Here's how the part is built. I have some questions about the finished solid (model axes, mm). Face numbers are marked on the shaded views. A direction names the side the tool comes from. Give positions to 0.01 mm unless a question says otherwise; leave off trailing zeros. Write each loop counter-clockwise with the first axis right and the second up, starting at its lowest first coordinate (ties: lowest second). Pieces come first, ordered by that corner, then holes. Notation, with made-up numbers: (42.5, 6.25) - (77.5, 6.25) arc R30 ccw to (77.5, 45.25) - close; hole circle Ø10 at (-17.75, 35.25). An arc over 180 degrees is marked (long way). Use a Markdown table: item, result.
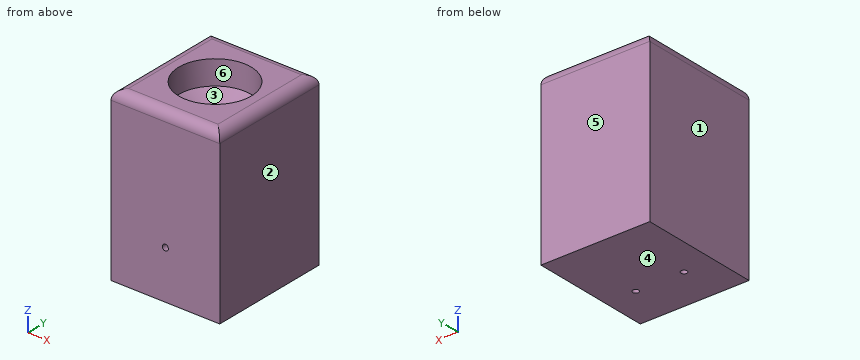
```python
from build123d import *

# Parameters (mm, degrees)
F0_W     = 57.15
F0_H     = 63.5
F1_DEPTH = 88.9
F3_D     = 38.1
F3_DEPTH = 12.7
F3_TIP   = 11.4463947925
F4_R     = 5.08
F6_D     = 3.175
F6_DEPTH = 12.7
F6_TIP   = 0.9538662327
F8_D     = 3.175


with BuildPart() as f1:
    # F0 (on Top) → F1 (new body)
    with BuildSketch(Plane.XY):
        with Locations((28.575, -31.75)):
            Rectangle(F0_W, F0_H)
    extrude(amount=F1_DEPTH)

    # F3
    with Locations(Plane.XY.offset(88.9)):
        with Locations((28.575, -31.75)):
            Hole(F3_D / 2, depth=F3_DEPTH)
            with Locations((0, 0, -(F3_DEPTH + F3_TIP / 2))):  # 118° drill point
                Cone(0, F3_D / 2, F3_TIP, mode=Mode.SUBTRACT)

    # F4
    f4_edges = [f1.edges().sort_by_distance(p)[0] for p in [
        (57.15, -31.75, 88.9),
        (28.575, 0, 88.9),
        (0, -31.75, 88.9),
        (28.575, -63.5, 88.9),
    ]]
    fillet(f4_edges, radius=F4_R)

    # F6
    with Locations(Plane.XZ.offset(63.5)):
        with Locations((28.575, 25.4)):
            Hole(F6_D / 2, depth=F6_DEPTH)
            with Locations((0, 0, -(F6_DEPTH + F6_TIP / 2))):  # 118° drill point
                Cone(0, F6_D / 2, F6_TIP, mode=Mode.SUBTRACT)

    # F8 (through all)
    with Locations(Plane(origin=(0, 0, 0), x_dir=(1, 0, 0), z_dir=(0, 0, -1))):
        with Locations((41.275, 41.275), (15.875, 41.275)):
            Hole(F8_D / 2)


solid = f1.part
```
Item 1: I need wall thicknesses on line 1 along X through (y, z) = (-57.5, 25.4); line 2 along X through (y, z) = (-31, 79); line 3 along X through (y, z) = (-40.5, 6). Which ranges of each line are inside material? Lowest first, please. Write a range as [from, to].
Values:
| item | result |
|---|---|
| line 1 | x = [0, 26.99], [30.16, 57.15] |
| line 2 | x = [0, 9.54], [47.61, 57.15] |
| line 3 | x = [0, 14.49], [17.26, 39.89], [42.66, 57.15] |
Item 2: If we section it at A-A, the plane z = 77.5: Write out the boundary of the cut face in (x, y) (3 decimals).
Values:
| item | result |
|---|---|
| outline | (0, -63.5) - (57.15, -63.5) - (57.15, 0) - (0, 0) - close; hole circle Ø38.1 at (28.575, -31.75) |
Item 3: For the marked faces 5 and 6, which set-ups out of +Z, -Z, +X, -X, +Y, -Y let a thin tool reach every point of the face, with its end or its side?
Values:
| item | result |
|---|---|
| face 5 | +Z, -Z, +X, -X, +Y |
| face 6 | +Z |
Item 4: Thinking about a two-plate mould opening in X: for the marked faces 1, 2, 3 and 4, which applies, +X half, -X half, draft (parallel to the pull), parting line (faces both ways), or undercut?
Values:
| item | result |
|---|---|
| face 1 | -X half |
| face 2 | +X half |
| face 3 | undercut |
| face 4 | draft |
